from build123d import *

# Parameters (mm, degrees)
F0_W     = 11
F0_H     = 30
F1_DEPTH = 24
F3_DEPTH = 11


# Not quite as in the source:
# - a feature of the source that left no trace in its solid (it failed there, or was rolled back) is left out


with BuildPart() as f1:
    # F0 (on Right) → F1 (new body, symmetric)
    with BuildSketch(Plane.YZ):
        with BuildLine():
            ThreePointArc((15.4919333848, 11), (18.1017503893, 5.7729223833), (19, 0))
            Line((19, 0), (30, 0))
            ThreePointArc((30, 0), (29.4730143031, 5.5983415304), (27.9105714739, 11))
            Line((27.9105714739, 11), (15.4919333848, 11))
        make_face()
        with BuildLine():
            ThreePointArc((-15.4919333848, 11), (0, 19), (15.4919333848, 11))
            Line((15.4919333848, 11), (27.9105714739, 11))
            ThreePointArc((27.9105714739, 11), (0, 30), (-27.9105714739, 11))
            Line((-27.9105714739, 11), (-15.4919333848, 11))
        make_face()
        with BuildLine():
            Line((-30, 0), (-19, 0))
            ThreePointArc((-19, 0), (-18.1017503893, 5.7729223833), (-15.4919333848, 11))
            Line((-15.4919333848, 11), (-27.9105714739, 11))
            ThreePointArc((-27.9105714739, 11), (-29.4730143031, 5.5983415304), (-30, 0))
        make_face()
        with BuildLine():
            ThreePointArc((27.9105714739, 11), (29.4730143031, 5.5983415304), (30, 0))
            Line((30, 0), (51, 0))
            Line((51, 0), (51, 11))
            Line((51, 11), (40, 11))
            Line((40, 11), (27.9105714739, 11))
        make_face()
        with BuildLine():
            Line((-56, 0), (-30, 0))
            ThreePointArc((-30, 0), (-29.4730143031, 5.5983415304), (-27.9105714739, 11))
            Line((-27.9105714739, 11), (-56, 11))
            Line((-56, 11), (-56, 0))
        make_face()
        with Locations((45.5, 26)):
            Rectangle(F0_W, F0_H)
    extrude(amount=F1_DEPTH, both=True)

    # F2 (on face) → F3 (cut, through all)
    with BuildSketch(Plane(origin=(0, 51, 0), x_dir=(-1, 0, 0), z_dir=(0, 1, 0))):
        with BuildLine():
            ThreePointArc((-6.5, 25), (0, 18.5), (6.5, 25))
            ThreePointArc((6.5, 25), (0, 31.5), (-6.5, 25))
        make_face()
        with BuildLine():
            ThreePointArc((-6.5, 25), (0, 31.5), (6.5, 25))
            Line((6.5, 25), (6.5, 41))
            Line((6.5, 41), (-6.5, 41))
            Line((-6.5, 41), (-6.5, 25))
        make_face()
    extrude(amount=-F3_DEPTH, mode=Mode.SUBTRACT)


solid = f1.part
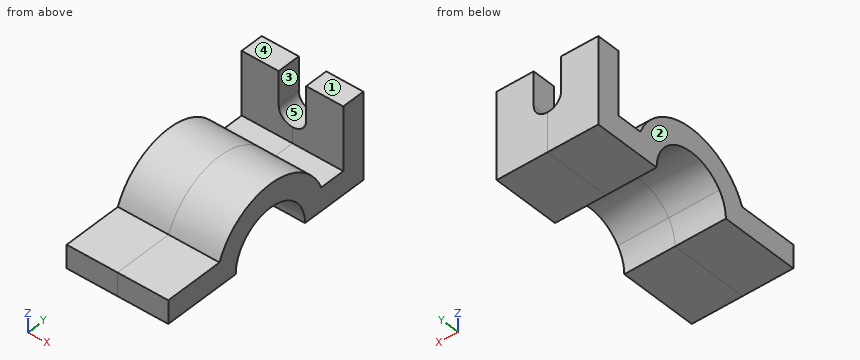
Verification items for the finished model (mm, model axes). Face numbers are marked on the shaded views. A direction names the side the tool comes from. Coordinates: 2 decimals unless noted, no trailing zeros. Write each loop counter-clockwise with the first axis right and the second up, starting at its lowest first coordinate (ties: lowest second). Pieces come first, ordered by that corner, then holes. Notation, with made-up numbers: (37, -40) - (56, -40) arc R21 cw to (56, -7) - close; hole circle Ø10 at (80.5, -23). An arc over 180 degrees is marked (long way). Answer as a JSON object with one key per item and string values.
(1) Mould release check, pull along X, two halves, no side actions. Record for the marked faces 1, 2 and 3: pulls with the +X half, pulls with the -X half, needs draft (parallel to the pull), parting line crosses it, or undercut.
Report:
{"face 1": "needs draft", "face 2": "pulls with the -X half", "face 3": "undercut"}
(2) Cross-section at A-A on z = 31.5. Record the cut outline in (x, y).
Report:
{"outline": "(-24, 40) - (-6.5, 40) - (-6.5, 51) - (-24, 51) - close; (6.5, 40) - (24, 40) - (24, 51) - (6.5, 51) - close"}
(3) Cross-section at C-C on x = 17.5. Record the cut outline in (y, z), plus the area to 3 significant figures.
Report:
{"outline": "(-56, 0) - (-19, 0) arc R19 cw to (19, 0) - (51, 0) - (51, 41) - (40, 41) - (40, 11) - (27.91, 11) arc R30 ccw to (-27.91, 11) - (-56, 11) - close", "area": "1,710 mm^2"}
(4) Thickness scan on line 1 along Y through (x, z) = (11, 12); line 2 along Y through (x, z) = (-9, 33.5); line 3 along Y through (x, z) = (-7, 16). Record the ranges inside material, lowest first.
Report:
{"line 1": "-27.5 to -14.73, 14.73 to 27.5, 40 to 51", "line 2": "40 to 51", "line 3": "-25.38 to -10.25, 10.25 to 25.38, 40 to 51"}
(5) Cross-section at B-B on z = 26. Record the cut outline in (x, y).
Report:
{"outline": "(-24, -14.97) - (24, -14.97) - (24, 14.97) - (-24, 14.97) - close; (-24, 40) - (-6.5, 40) - (-6.5, 51) - (-24, 51) - close; (6.5, 40) - (24, 40) - (24, 51) - (6.5, 51) - close"}
(6) Tool access check on the marked faces 4 and 5. Record the directions out of +Z, -Z, +X, -X, +Y, -Y that give a thin tool (end or side, any length) a straight path to the whole face; none if there is none.
Report:
{"face 4": "+Z, +X, -X, +Y, -Y", "face 5": "+Z, +Y"}
(7) Gauge pin test, flat ends, axial feed: pin 1 Ø7 at (x, z) = (-13.5, 29.5) entering from -Y; pin 2 Ø5 at (x, y) = (7, 17.5) entering from +Z; pin 3 Ø7 at (x, z) = (16.5, 19) entering from -Y. Record the tip position at first contact, or that the pin passes through.
Report:
{"pin 1": "y = -14.97", "pin 2": "z = 25.98", "pin 3": "y = -25.69"}
(8) Cross-section at D-D on y = 43. Record the cut outline in (x, z), plus the area to 3 significant figures.
Report:
{"outline": "(-24, 0) - (24, 0) - (24, 41) - (6.5, 41) - (6.5, 25) arc R6.5 cw to (-6.5, 25) - (-6.5, 41) - (-24, 41) - close", "area": "1,690 mm^2"}
